Source: CAD feature listing. Evaluate the final solid. Frame: model axes, mm. Face numbers are marked on the shaded views. A direction names the side the tool comes from. Coordinates: 2 decimals unless noted, no trailing zeros. Order: outer loops, then holes, each group sorted by start corner. A loop starts at its lowest first (then second) coordinate and runs counter-clockwise, first axis right, second up.
Autodesk Inventor part; units mm, degrees
ref_plane "YZ Plane" through (0, 0, 0) normal (1, 0, 0) x (0, 1, 0)
ref_plane "XZ Plane" through (0, 0, 0) normal (0, 1, 0) x (-1, 0, 0)
ref_plane "XY Plane" through (0, 0, 0) normal (0, 0, 1) x (1, 0, 0)
sketch "Sketch1" plane through (0, 0, 0) normal (0, 1, 0) x (-1, 0, 0)
  line L0 (0, 0) -> (-143, 0)
  line L1 (-143, 0) -> (-143, 73)
  line L2 (-143, 73) -> (0, 73)
  line L3 (0, 73) -> (0, 0)
  line L4 (-38.5547, 3.9462) -> (-41.5547, 3.9462)
  circle A0 centre (-19, 19) radius 16
  circle A1 centre (-54, 19) radius 16
  circle A2 centre (-89, 19) radius 16
  circle A3 centre (-124, 19) radius 16
  circle A4 centre (-124, 54) radius 16
  circle A5 centre (-89, 54) radius 16
  circle A6 centre (-54, 54) radius 16
  circle A7 centre (-19, 54) radius 16
  dimension "d10" = 3
  dimension "d12" = 32
  dimension "d13" = 32
  dimension "d14" = 32
  dimension "d15" = 32
  dimension "d16" = 32
  dimension "d17" = 32
  dimension "d18" = 32
  dimension "d19" = 32
  dimension "d20" = 35
  dimension "d21" = 19
  dimension "d22" = 35
  dimension "d23" = 35
  dimension "d24" = 19
  dimension "d25" = 19
  dimension "d26" = 19
  dimension "d27" = 19
  dimension "d28" = 19
  dimension "d29" = 19
  dimension "d30" = 35
  dimension "d31" = 35
  dimension "d32" = 35
  dimension "d33" = 35
  dimension "d34" = 19
extrude "Extrusion1" add sketch "Sketch1" against normal blind 70
sketch "Sketch3" plane through (143, 0, 0) normal (0, 0, -1) x (-1, 0, 0)
  line L0 (138, -65) -> (5, -65)
  line L1 (5, -65) -> (5, -38)
  line L2 (5, -38) -> (138, -38)
  line L3 (138, -38) -> (138, -65)
  line L4 (143, 0) -> (143, -70)
  line L5 (0, 0) -> (0, -70)
  line L6 (143, -70) -> (0, -70)
  line L7 (0, 0) -> (143, 0)
  line L8 (5, -5) -> (138, -5)
  line L9 (138, -5) -> (138, -33)
  line L10 (138, -33) -> (5, -33)
  line L11 (5, -33) -> (5, -5)
  line L12 (5, -5) -> (138, -33) construction
  line L13 (138, -5) -> (5, -33) construction
  point P0 (71.5, -19)
  dimension "d37" = 5
  dimension "d38" = 5
  dimension "d39" = 5
  dimension "d57" = 5
  dimension "d58" = 5
  dimension "d59" = 5
  dimension "d63" = 5
extrude "Extrusion2" cut sketch "Sketch3" against normal through all contours L0 L1 L2 L3 | L8 L9 L10 L11
sketch "Sketch4" plane through (0, 0, 0) normal (-1, 0, 0) x (0, 0, 1)
  line L0 (5, -5) -> (68, -5)
  line L1 (68, -5) -> (68, -33)
  line L2 (68, -33) -> (5, -33)
  line L3 (5, -33) -> (5, -5)
  line L4 (0, 0) -> (73, 0)
  line L5 (0, 0) -> (0, -70)
  line L6 (73, 0) -> (73, -70)
  line L7 (5, -38) -> (68, -38)
  line L8 (68, -38) -> (68, -65)
  line L9 (68, -65) -> (5, -65)
  line L10 (5, -65) -> (5, -38)
  line L11 (73, -70) -> (0, -70)
  dimension "d45" = 5
  dimension "d46" = 5
  dimension "d47" = 5
  dimension "d49" = 5
  dimension "d50" = 5
  dimension "d51" = 5
  dimension "d62" = 5
extrude "Extrusion3" cut sketch "Sketch4" against normal through all contours L0 L1 L2 L3 | L7 L8 L9 L10
sketch "Sketch5" plane through (0, -70, 0) normal (0, -1, 0) x (1, 0, 0)
  line L0 (143, 0) -> (0, 0)
  line L1 (143, 0) -> (0, 0)
  line L2 (0, 0) -> (0, 73)
  line L3 (0, 73) -> (143, 73)
  line L4 (143, 73) -> (143, 0)
extrude "Extrusion4" add sketch "Sketch5" against normal blind 3
equation "\"d13\" = d12"
equation "\"d14\" = d12"
equation "\"d15\" = d12"
equation "\"d16\" = d12"
equation "\"d17\" = d12"
equation "\"d18\" = d12"
equation "\"d19\" = d12"
equation "\"d20\" = d12 + d10"
equation "\"d21\" = 0.5 * d12 + d10"
equation "\"d22\" = d20"
equation "\"d24\" = d21"
equation "\"d25\" = d21"
equation "\"d26\" = d21"
equation "\"d27\" = d25"
equation "\"d28\" = d27"
equation "\"d30\" = d20"
equation "\"d32\" = d31"
equation "\"d34\" = d29"
equation "\"d38\" = d37"
equation "\"d39\" = d37"
equation "\"d57\" = d37"
equation "\"d58\" = d38"
equation "\"d59\" = d37"
equation "\"d63\" = d37"
equation "\"d46\" = d45"
equation "\"d47\" = d45"
equation "\"d49\" = d45"
equation "\"d50\" = d45"
equation "\"d51\" = d45"
equation "\"d62\" = d45"
properties part number "falcon tube mount v01"
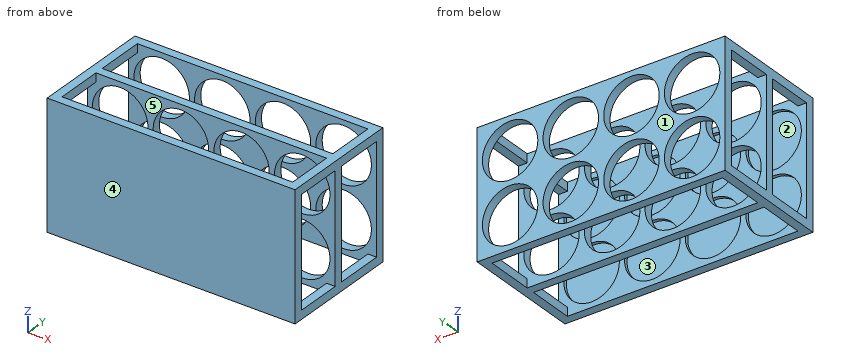
1. Access query for the marked faces 1 and 2. Directions: +Z, -Z, +X, -X, +Y, -Y. A direction counts if a zero-diameter tool reaches every point of the face in a straight line with its end or side. Return the directions, or none.
2. Draft query along Y for the marked faces 3, 4 and 5. Return one class per face: +Y half, -Y half, draft (parallel to the pull), parting line (faces both ways), or undercut.
3. Section query B-B, the plane x = 19. Count the separate pieces of the cut face and the enclosed holes in it, plus the area to 3 significant figures.
4. Section query A-A, the plane y = -19.5. Output: boundary loops of the cut face in (x, z), plus the area to 3 significant figures.
5. Material intervals for line 1 along Z through (x, y) = (124, -2.25); line 2 along X through (y, z) = (-36.45, 19); line 3 along Y through (x, z) = (38, 31), sorted ascending.
Answer key:
1. face 1: +Z, -Z, +X, -X, +Y
1. face 2: +Y
2. face 3: +Y half
2. face 4: -Y half
2. face 5: undercut
3. separate pieces: 7
3. enclosed holes: 0
3. area: 327 mm2
4. outline: (0, 0) - (5, 0) - (5, 5) - (0, 5) - close; (0, 68) - (5, 68) - (5, 73) - (0, 73) - close; (138, 0) - (143, 0) - (143, 5) - (138, 5) - close; (138, 68) - (143, 68) - (143, 73) - (138, 73) - close
4. area: 100 mm2
5. line 1: z = 0 to 3, 35 to 38, 70 to 73
5. line 2: x = 0 to 3, 35 to 38, 70 to 73, 105 to 108, 140 to 143
5. line 3: y = -70 to -65, -38 to -33, -5 to 0
